Geometry check sheet. Reference: drawing and pictorial views, mm from the part's lowest x, y, z. A direction names the side the tool comes from. Coordinates: 2 decimals unless noted, no trailing zeros. Write each loop counter-clockwise with the first axis right and the second up, starting at its lowest first coordinate (ties: lowest second). Pieces come first, ordered by that corner, then holes. Notation, with made-up numbers: (-28.75, 75) - (-10.75, 75) arc R18 ccw to (-10.75, 84) - close; hole circle Ø4 at (81, -37.75). An arc over 180 degrees is marked (long way). Use one line per item in the form item = value. Start each with the question number.
(1) Material ranges on line 1 (X direction, y = 20, z = 1.25); line 2 (Z direction, x = 183, y = 4); line 3 (X direction, y = 33, z = 6.75), recorded low to high. Write a range as [from, to].
(2) Sectioned sample at D-D (x = 98.5). Record the cut outline in (y, z), and give its area (3 significant figures).
(3) Gauge pin test, flat ends, axial feed: pin 1 Ø2 at (x, y) = (131.5, 9) entering from +Z; pin 2 Ø1 at (x, y) = (172, 24) entering from +Z; pin 3 Ø2.5 at (x, z) = (73, 6.5) entering from -Y. Record the tip position at first contact, or that the pin passes through.
(4) Tool access check on the marked faces 1 and 2. Record the directions out of +Z, -Z, +X, -X, +Y, -Y that give a thin tool (end or side, any length) a straight path to the whole face; none if there is none.
(5) Sectioned sample at B-B (y = 12). Record the cut outline in (x, z), and give its area (3 significant figures).
(6) Sectioned sample at A-A (z = 7.5). Record the cut outline in (x, y), and give its area (3 significant figures).
(7) Sectioned sample at C-C (y = 27.5). Record the cut outline in (x, z), and give its area (3 significant figures).
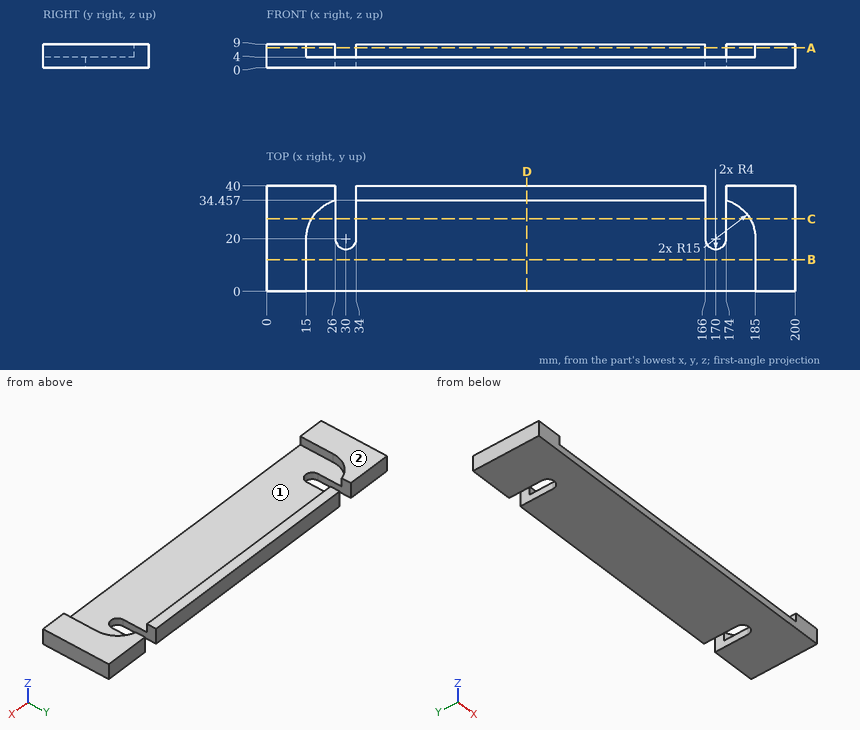
Answers below:
q1.line_1 = [0, 26], [34, 166], [174, 200]
q1.line_2 = [0, 4]
q1.line_3 = [0, 22.52], [177.48, 200]
q2.outline = (0, 0) - (40, 0) - (40, 9) - (34.46, 9) - (34.46, 4) - (0, 4) - close
q2.area = 188 mm2
q3.pin_1 = 4
q3.pin_2 = through
q3.pin_3 = 34.46
q4.face_1 = +Z, -Y
q4.face_2 = +Z, +X, -X, +Y, -Y
q5.outline = (0, 0) - (200, 0) - (200, 9) - (185, 9) - (185, 4) - (15, 4) - (15, 9) - (0, 9) - close
q5.area = 950 mm2
q6.outline = (0, 0) - (15, 0) - (15, 20) arc R15 cw to (26, 34.46) - (26, 40) - (0, 40) - close; (34, 34.46) - (166, 34.46) - (166, 40) - (34, 40) - close; (174, 34.46) arc R15 cw to (185, 20) - (185, 0) - (200, 0) - (200, 40) - (174, 40) - close
q6.area = 2,140 mm2
q7.outline = (0, 0) - (26, 0) - (26, 4) - (17.01, 4) - (17.01, 9) - (0, 9) - close; (34, 0) - (166, 0) - (166, 4) - (34, 4) - close; (174, 0) - (200, 0) - (200, 9) - (182.99, 9) - (182.99, 4) - (174, 4) - close
q7.area = 906 mm2
